The listing builds one solid part. Answer for the finished solid, in the listing's coordinates (mm). Face numbers are marked on the shaded views. A direction names the side the tool comes from. Round coordinates to 2 decimals unless told otherwise and drop trailing zeros. Order: outer loops, then holes, each group sorted by start corner. A loop starts at its lowest first (then second) coordinate and runs counter-clockwise, first axis right, second up. Notation, with made-up numbers: M -35,36.5 L -11,36.5 A21 ccw -11,49.5 Z; hole C 54.25,87.5 d7. An arc over 180 degrees is marked long. Put each result on its own line as item: value. Start each with the question number.
1. The part is cut by section A-A (x = 330). Give the vertices of the cut face in (y, z), then the cut area to 3 significant figures.
2. Consider line 1 (Z direction, x = 251, y = -16.5); line 2 (Y direction, x = 615.5, z = -3); line 3 (Z direction, x = 596.5, y = -25). Determine where each line is inside the solid, lowest interval first.
3. Which of the six approach directions +Z, -Z, +X, -X, +Y, -Y give full straight-line access (tool end or side, diameter ignored) to the marked faces 1 and 2?
4. The part is cut by section B-B (y = -2). Give the vertices of the cut face in (x, z).
5. The part is cut by section C-C (z = 25.5). Give the vertices of the cut face in (x, y).
6. Each of these flat-tipped pins is pushed along its axis until it touches: pin 1 Ø5 at (x, z) = (476.5, 10) entering from +Y; pin 2 Ø5 at (x, y) = (384.5, 10) entering from -Z. Where does it stop, or does it pass through?
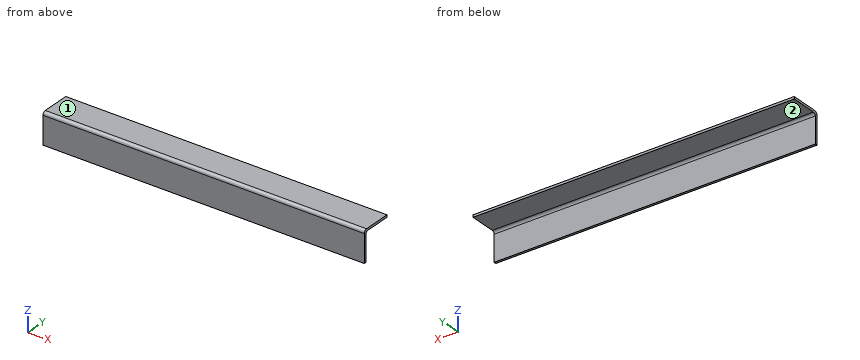
from build123d import *

# Parameters (mm, degrees)
F1_DEPTH = 660.4


with BuildPart() as f1:
    # F0 (on Right) → F1 (new body)
    with BuildSketch(Plane.YZ):
        with BuildLine():
            Line((-28.115756, 44.895094), (-28.115756, -12.254906))
            Line((-28.115756, -12.254906), (-23.353256, -12.254906))
            Line((-23.353256, -12.254906), (-23.353256, 41.402594))
            ThreePointArc((-23.353256, 41.402594), (-21.865359, 44.994697), (-18.273256, 46.482594))
            Line((-18.273256, 46.482594), (35.384244, 46.482594))
            Line((35.384244, 46.482594), (35.384244, 51.245094))
            Line((35.384244, 51.245094), (-21.765756, 51.245094))
            ThreePointArc((-21.765756, 51.245094), (-26.255884, 49.385222), (-28.115756, 44.895094))
        make_face()
    extrude(amount=F1_DEPTH)


solid = f1.part
Resolved:
1. outline: M -28.12,-12.25 L -23.35,-12.25 L -23.35,41.4 A5.08 cw -18.27,46.48 L 35.38,46.48 L 35.38,51.25 L -21.77,51.25 A6.35 ccw -28.12,44.9 Z
1. area: 579 mm2
2. line 1: 46.48 to 51.25
2. line 2: -28.12 to -23.35
2. line 3: -12.25 to 50.36
3. face 1: +Z, +X, -X, +Y, -Y
3. face 2: -Z, +X, -X, +Y
4. outline: M 0,46.48 L 660.4,46.48 L 660.4,51.25 L 0,51.25 Z
5. outline: M 0,-28.12 L 660.4,-28.12 L 660.4,-23.35 L 0,-23.35 Z
6. pin 1: y = -23.35
6. pin 2: z = 46.48
